from build123d import *

# Parameters (mm, degrees)
SKETCH1_R           = 0.25
BOSS_EXTRUDE1_DEPTH = 2
SWEEP1_OUTLINE_R    = 0.25
SWEEP1_DEPTH        = 2.5
SWEEP1_2_OUTLINE_R  = 0.25
SWEEP1_2_ANGLE      = 90
SWEEP1_3_OUTLINE_R  = 0.25
SWEEP1_3_ANGLE      = 90
SWEEP1_START        = 0.4999999
SWEEP1_4_OUTLINE_R  = 0.25
SWEEP1_4_DEPTH      = 30.2000002


with BuildPart() as part:
    # Sketch1 → Boss-Extrude1 (new body)
    with BuildSketch(Plane(origin=(0, 0, 0), x_dir=(1, 0, 0), z_dir=(0, 1, 0))):
        with Locations(Location((0, 0, 0), (0, 0, 270))):
            Circle(SKETCH1_R)
    extrude(amount=BOSS_EXTRUDE1_DEPTH)

    # Sweep1: read off the stored shape, not the designer's step
    # Sweep1 outline → Sweep1 (add)
    with BuildSketch(Plane(origin=(0, 0, 0), x_dir=(1, 0, 0), z_dir=(0, 1, 0))):
        Circle(SWEEP1_OUTLINE_R)
        with Locations((31.2, 0)):
            Circle(SWEEP1_OUTLINE_R)
    extrude(amount=SWEEP1_DEPTH)

    # Sweep1 2 outline → Sweep1 2 (revolve)
    with BuildSketch(Plane(origin=(0.5, 2.5, 0), x_dir=(0, 1, 0), z_dir=(1, 0, 0))):
        with Locations((0.5, 0)):
            Circle(SWEEP1_2_OUTLINE_R)
    revolve(axis=Axis((0.5, 2.5, 0), (0, 0, 1)), revolution_arc=SWEEP1_2_ANGLE)

    # Sweep1 3 outline → Sweep1 3 (revolve)
    with BuildSketch(Plane(origin=(30.7, 2.5, 0), x_dir=(1, 0, 0), z_dir=(0, -1, 0))):
        with Locations((0.5, 0)):
            Circle(SWEEP1_3_OUTLINE_R)
    revolve(axis=Axis((30.7, 2.5, 0), (0, 0, 1)), revolution_arc=SWEEP1_3_ANGLE)

    # Sweep1 4 outline → Sweep1 4 (add)
    with BuildSketch(Plane.YZ.offset(SWEEP1_START)):
        with Locations((3, 0)):
            Circle(SWEEP1_4_OUTLINE_R)
    extrude(amount=SWEEP1_4_DEPTH)


solid = part.part
Can you work these out from the model? Positions are in its coordinate system, mm. Give positions to 0.01 mm unless a question says otherwise; leave off trailing zeros. Write each loop counter-clockwise with the first axis right and the second up, starting at its lowest first coordinate (ties: lowest second). Pieces come first, ordered by that corner, then holes. Notation, with made-up numbers: (53, 88.5) -> (85, 88.5) arc R10 cw to (85, 106.5) -> close; hole circle Ø1 at (27.5, -29). An arc over 180 degrees is marked (long way). Answer as a JSON object with one key per item and string values. Group by question number.
Item 1: Suppose I cut it at B-B (x = 21). Please give me the cut outline in (y, z).
Item 2: Suppose I cut it at C-C (z = -0.1). Please give me the cut outline in (x, y), plus the area to 3 significant figures.
Item 3: Suppose I cut it at A-A (y = 1.05). Please give me the cut outline in (x, z).
Item 4: Please list where these lines run through material, in increasing order: line 1 (X direction, y = 0.35, z = 0.05); line 2 (Z direction, x = 11.5, y = 3.05); line 3 (X direction, y = 1.95, z = 0.2). Write a range as [from, to].
Findings:
{
 "1": {"outline": "circle Ø0.5 at (3, 0)"},
 "2": {"outline": "(-0.23, 0) -> (0.23, 0) -> (0.23, 2.5) arc R0.27 cw to (0.5, 2.77) -> (30.7, 2.77) arc R0.27 cw to (30.97, 2.5) -> (30.97, 0) -> (31.43, 0) -> (31.43, 2.5) arc R0.73 ccw to (30.7, 3.23) -> (0.5, 3.23) arc R0.73 ccw to (-0.23, 2.5) -> close", "area": "16.9 mm²"},
 "3": {"outline": "circle Ø0.5 at (0, 0); circle Ø0.5 at (31.2, 0)"},
 "4": {"line 1": "x = [-0.24, 0.24], [30.96, 31.44]", "line 2": "z = [-0.24, 0.24]", "line 3": "x = [-0.15, 0.15], [31.05, 31.35]"}
}
